For this review, use the dimensioned drawing (mm, ordinates from the lowest corner) and the shaded views. A direction names the side the tool comes from. Coordinates: 2 decimals unless noted, no trailing zeros. Order: outer loops, then holes, each group sorted by start corner. A loop starts at its lowest first (then second) coordinate and runs counter-clockwise, first axis right, second up. Notation, with made-up numbers: M -25.75,69 L -12.75,69 A15 cw -12.75,84 Z; hole C 5,14 d8. An arc over 180 degrees is marked long. Answer as CSV lines item,"result". Start each with the question number.
Q1. Consider section C-C on y = 2.5. Write out the cut boundary in (x, z).
Q2. Consider section B-B on z = 0.5. Write out the cut boundary in (x, y).
Q3. Wall thickness on L1, parallel to X at y = 1.75, z = 3.25; L2, parallel to Y at x = 15, z = 1.3; L3, parallel to Z at x = 17.25, y = 18.5: over which ranges is each line inside the solid? List them lowest first. Write a range as [from, to].
Q4. The part is to be moulded in two halves that separate along Y. For the marked faces 4, 5, 6 and 7, say which applies: +Y half, -Y half, draft (parallel to the pull), parting line (faces both ways), or undercut.
Q5. Consider section A-A on x = 15. Write out the cut boundary in (y, z).
Q6. For P1, Ø11, axis at x = 16.5, y = 16.5, coming from the +Z side; P2, Ø2, axis at x = 7, z = 1.5, coming from the -Y side; P3, Ø2, axis at y = 13.5, z = 1.5, coming from the -X side, all flat-tipped, find the tip position at first contact; note any pin that passes through.
Q7. Machinability: for the marked faces 1, 2 and 3, which of the approach directions +Z, -Z, +X, -X, +Y, -Y give a long, thin tool a straight path to every point of the face, cutting with its end or side? Answer none if there is none.
Q8. Consider section D-D on y = 17.5. Write out the cut boundary in (x, z).
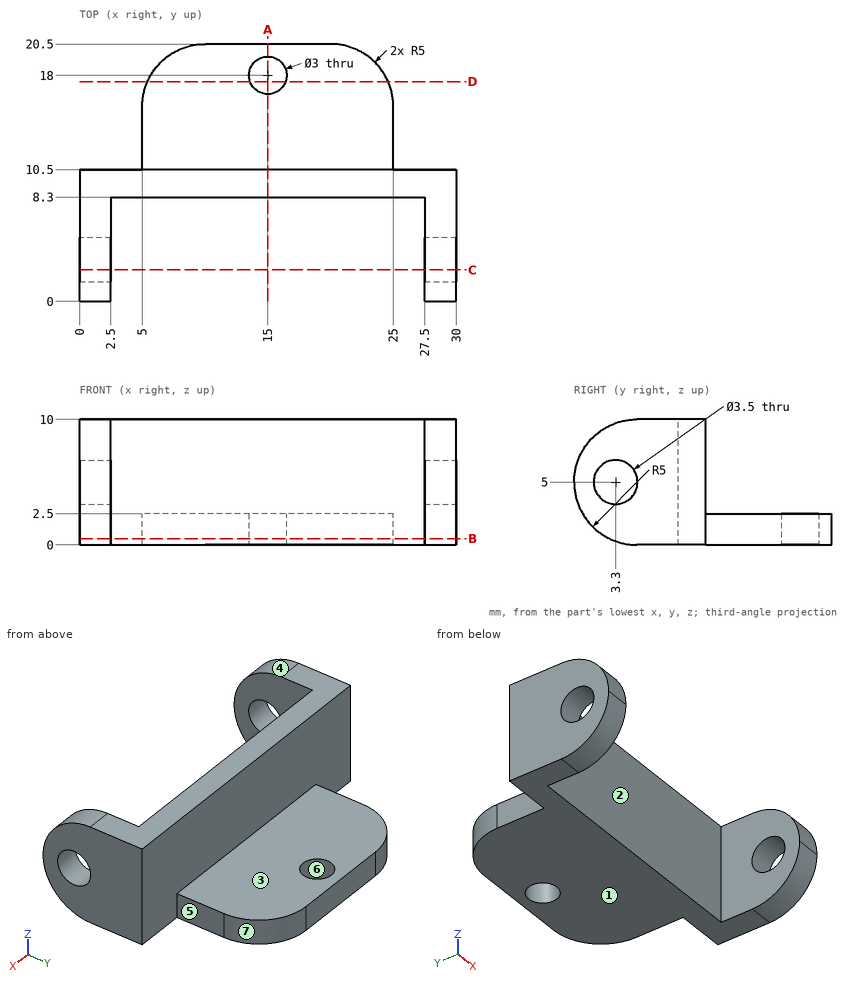
Evaluation:
1,outline,"M 0,0.67 L 2.5,0.67 L 2.5,3.44 L 0,3.44 Z; M 0,6.56 L 2.5,6.56 L 2.5,9.33 L 0,9.33 Z; M 27.5,0.67 L 30,0.67 L 30,3.44 L 27.5,3.44 Z; M 27.5,6.56 L 30,6.56 L 30,9.33 L 27.5,9.33 Z"
2,outline,"M 0,2.82 L 2.5,2.82 L 2.5,8.3 L 27.5,8.3 L 27.5,2.82 L 30,2.82 L 30,10.5 L 25,10.5 L 25,15.5 A5 ccw 20,20.5 L 10,20.5 A5 ccw 5,15.5 L 5,10.5 L 0,10.5 Z; hole C 15,18 d3"
3,L1,"x = [0, 2.5], [27.5, 30]"
3,L2,"y = [8.3, 16.5], [19.5, 20.5]"
3,L3,"z = [0, 2.5]"
4,face 4,"-Y half"
4,face 5,"draft"
4,face 6,"undercut"
4,face 7,"+Y half"
5,outline,"M 8.3,0 L 16.5,0 L 16.5,2.5 L 10.5,2.5 L 10.5,10 L 8.3,10 Z; M 19.5,0 L 20.5,0 L 20.5,2.5 L 19.5,2.5 Z"
6,P1,"stops at z = 2.5"
6,P2,"stops at y = 8.3"
6,P3,"stops at x = 5"
7,face 1,"-Z, +X, -X, +Y, -Y"
7,face 2,"+Z, -Z, -Y"
7,face 3,"+Z, +X, -X, +Y"
8,outline,"M 5.42,0 L 13.59,0 L 13.59,2.5 L 5.42,2.5 Z; M 16.41,0 L 24.58,0 L 24.58,2.5 L 16.41,2.5 Z"
